Can you work these out from the model? Positions are in its coordinate system, mm. Give positions to 0.01 mm unless a question says otherwise; leave off trailing zeros. Order: outer loops, then holes, each group sorted by start corner. A loop starts at its lowest first (then second) coordinate and runs counter-clockwise, first axis right, second up. Notation, with made-up numbers: (26.5, 31.5) - (74.5, 31.5) arc R28 cw to (74.5, 51.5) - close; hole circle Ø6 at (-10, -35.75). An arc over 180 degrees is marked (long way). Answer as CSV lines item,"result".
```python
from build123d import *

# Parameters (mm, degrees)
BOSS_EXTRUDE1_DEPTH     = 5
CUT_EXTRUDE1_DEPTH      = 57
CUT_EXTRUDE1_DEPTH_BACK = 57
SKETCH2_R               = 3
SKETCH3_W               = 140
SKETCH3_H               = 20
CUT_EXTRUDE2_DEPTH      = 10


with BuildPart() as part:
    # Sketch1 → Boss-Extrude1 (new body)
    with BuildSketch(Plane(origin=(0, 0, 0), x_dir=(1, 0, 0), z_dir=(0, 1, 0))):
        Polygon((0, -45), (21, -45), (21, -21), (45, -21), (45, 0), (295, 0), (295, -21), (319, -21), (319, -45), (340, -45), (340, -295), (319, -295), (319, -319), (295, -319), (295, -340), (45, -340), (45, -319), (21, -319), (21, -295), (0, -295), align=None)
    extrude(amount=BOSS_EXTRUDE1_DEPTH)

    # Sketch2 → Cut-Extrude1 (cut, two sides: drawn at the far end of the back side and taken through both)
    with BuildSketch(Plane(origin=(0, 5, 0), x_dir=(1, 0, 0), z_dir=(0, 1, 0)).offset(-CUT_EXTRUDE1_DEPTH_BACK)):
        with Locations(Location((75, -10, 0), (0, 0, 270))):
            Circle(SKETCH2_R)
        with Locations(Location((265, -10, 0), (0, 0, 270))):
            Circle(SKETCH2_R)
        with Locations(Location((265, -330, 0), (0, 0, 270))):
            Circle(SKETCH2_R)
        with Locations(Location((75, -330, 0), (0, 0, 270))):
            Circle(SKETCH2_R)
        with Locations(Location((10, -240, 0), (0, 0, 270))):
            Circle(SKETCH2_R)
        with Locations(Location((10, -100, 0), (0, 0, 270))):
            Circle(SKETCH2_R)
        with Locations(Location((330, -240, 0), (0, 0, 270))):
            Circle(SKETCH2_R)
        with Locations(Location((330, -100, 0), (0, 0, 270))):
            Circle(SKETCH2_R)
    extrude(amount=CUT_EXTRUDE1_DEPTH + CUT_EXTRUDE1_DEPTH_BACK, mode=Mode.SUBTRACT)

    # Sketch3 → Cut-Extrude2 (cut)
    with BuildSketch(Plane(origin=(0, 5, 0), x_dir=(1, 0, 0), z_dir=(0, 1, 0))):
        with Locations((170, -10)):
            Rectangle(SKETCH3_W, SKETCH3_H)
        with Locations((170, -330)):
            Rectangle(SKETCH3_W, SKETCH3_H)
    extrude(amount=-CUT_EXTRUDE2_DEPTH, mode=Mode.SUBTRACT)


solid = part.part
```
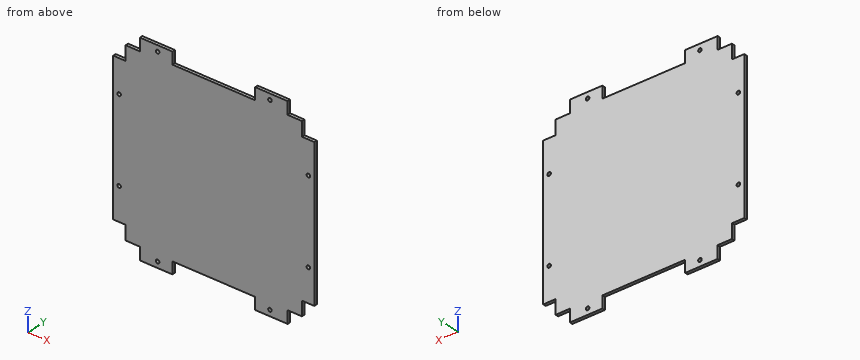
1) I want a section at A-A on y = 2.35. Count the separate pieces of the cut face and the enclosed holes in it, plus the area to 3 significant figures.
Answer block:
separate pieces,"1"
enclosed holes,"8"
area,"104,000 mm2"
2) I need wall thicknesses on line 1 along Z through (x, y) = (10, 1.9); line 2 along Z through (x, y) = (265, 3.1). Which ranges of each line are inside material? Lowest first, please. Write a range as [from, to].
Answer block:
line 1,"[45, 97], [103, 237], [243, 295]"
line 2,"[0, 7], [13, 327], [333, 340]"
3) I'm going to push flat-ended pins straight in: P1, Ø2, axis at x = 226.5, y = 1.5, coming from the +Z side; P2, Ø1.5, axis at x = 196, y = 2, coming from the -Z side; P3, Ø1.5, axis at y = 1.5, z = 325, coming from the -X side. Where does each tip first touch, or does it pass through?
Answer block:
P1,"z = 320"
P2,"z = 20"
P3,"x = 45"
4) I want a section at B-B on x = 157. Write out the boundary of the cut face in (y, z), plus the area to 3 significant figures.
Answer block:
outline,"(0, 20) - (5, 20) - (5, 320) - (0, 320) - close"
area,"1,500 mm2"
